from build123d import *

# Parameters (mm, degrees)
F0_W     = 292.1
F0_H     = 38.1
F1_DEPTH = 1219.2
F3_DEPTH = 1219.2
F4_W     = 12.7
F4_H     = 50.8
F5_DEPTH = 254


with BuildPart() as f1:
    # F0 (on Front) → F1 (new body)
    with BuildSketch(Plane.XZ):
        with Locations((146.05, 19.05)):
            Rectangle(F0_W, F0_H)
    extrude(amount=F1_DEPTH)

    # F2 (on face) → F3 (join)
    with BuildSketch(Plane.XZ.offset(1219.2)):
        with BuildLine():
            ThreePointArc((0, 41.275), (0.929936, 39.029936), (3.175, 38.1))
            Line((3.175, 38.1), (22.225, 38.1))
            ThreePointArc((22.225, 38.1), (24.470064, 39.029936), (25.4, 41.275))
            Line((25.4, 41.275), (25.4, 60.325))
            ThreePointArc((25.4, 60.325), (24.470064, 62.570064), (22.225, 63.5))
            Line((22.225, 63.5), (3.175, 63.5))
            ThreePointArc((3.175, 63.5), (0.929936, 62.570064), (0, 60.325))
            Line((0, 60.325), (0, 41.275))
        make_face()
        with BuildLine():
            ThreePointArc((22.6568, 41.275), (22.530329, 40.969671), (22.225, 40.8432))
            Line((22.225, 40.8432), (3.175, 40.8432))
            ThreePointArc((3.175, 40.8432), (2.869671, 40.969671), (2.7432, 41.275))
            Line((2.7432, 41.275), (2.7432, 60.325))
            ThreePointArc((2.7432, 60.325), (2.869671, 60.630329), (3.175, 60.7568))
            Line((3.175, 60.7568), (22.225, 60.7568))
            ThreePointArc((22.225, 60.7568), (22.530329, 60.630329), (22.6568, 60.325))
            Line((22.6568, 60.325), (22.6568, 41.275))
        make_face(mode=Mode.SUBTRACT)
    extrude(amount=-F3_DEPTH)

    # F4 (on face) → F5 (join)
    with BuildSketch(Plane(origin=(0, 0, 0), x_dir=(1, 0, 0), z_dir=(0, 0, -1))):
        with Locations((95.25, 1193.8)):
            Rectangle(F4_W, F4_H)
        with Locations((234.95, 1193.8)):
            Rectangle(F4_W, F4_H)
        with Locations((95.25, 838.2)):
            Rectangle(F4_W, F4_H)
        with Locations((234.95, 838.2)):
            Rectangle(F4_W, F4_H)
    extrude(amount=F5_DEPTH)


solid = f1.part
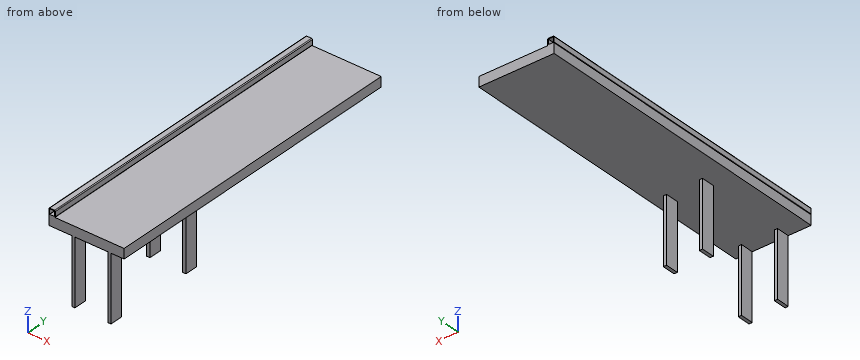
Could you check a few things on this model? Use its own coordinates, in mm. Coordinates: 2 decimals unless noted, no trailing zeros. Write each loop counter-clockwise with the first axis right and the second up, starting at its lowest first coordinate (ties: lowest second). Pieces come first, ordered by that corner, then holes. Notation, with made-up numbers: (24.5, -1) - (40.5, -1) arc R23 cw to (40.5, 18) - close; hole circle Ø2 at (-24.75, 80.5). An arc over 180 degrees is marked (long way). Put each result on its own line as item: value. Start each with the question number.
Q1. I'm going to push flat-ended pins straight in: P1, Ø10, axis at x = 221.5, z = 3, coming from the +Y side; P2, Ø6, axis at x = 95, z = -33, coming from the +Y side; P3, Ø15, axis at y = -838.5, z = -173, coming from the -X side; P4, Ø12, axis at x = 100.5, y = -979, coming from the +Z side. Where does each tip first touch, or does it pass through?
Q2. I want a section at C-C on x = 188.5. Write out the boundary of the cut face in (y, z), plus the area to 3 significant figures.
Q3. I want a section at A-A on z = -177. Write out the boundary of the cut face in (x, y), plus the area to 3 significant figures.
Q4. I want a section at B-B on y = -847. Write out the boundary of the cut face in (x, z) (3 decimals), plus the area to 3 significant figures.
Q5. Please list where these lines run through material, in increasing order: L1, parallel to X at y = -128.5, z = 41; L2, parallel to X at y = -996.5, z = 50.5; L3, parallel to Z at x = 180.5, y = -608.5.
Q6. I want a section at D-D on y = -457.5. Write out the boundary of the cut face in (x, z) (3 decimals), plus the area to 3 significant figures.
Checks:
1. P1: y = 0
1. P2: y = -812.8
1. P3: x = 88.9
1. P4: z = 38.1
2. outline: (-1219.2, 0) - (0, 0) - (0, 38.1) - (-1219.2, 38.1) - close
2. area: 46,500 mm²
3. outline: (88.9, -1219.2) - (101.6, -1219.2) - (101.6, -1168.4) - (88.9, -1168.4) - close; (88.9, -863.6) - (101.6, -863.6) - (101.6, -812.8) - (88.9, -812.8) - close; (228.6, -1219.2) - (241.3, -1219.2) - (241.3, -1168.4) - (228.6, -1168.4) - close; (228.6, -863.6) - (241.3, -863.6) - (241.3, -812.8) - (228.6, -812.8) - close
3. area: 2,580 mm²
4. outline: (0, 0) - (88.9, 0) - (88.9, -254) - (101.6, -254) - (101.6, 0) - (228.6, 0) - (228.6, -254) - (241.3, -254) - (241.3, 0) - (292.1, 0) - (292.1, 38.1) - (22.225, 38.1) arc R3.175 ccw to (25.4, 41.275) - (25.4, 60.325) arc R3.175 ccw to (22.225, 63.5) - (3.175, 63.5) arc R3.175 ccw to (0, 60.325) - (0, 41.275) arc R3.175 ccw to (3.175, 38.1) - (0, 38.1) - close; hole (2.743, 41.275) arc R0.432 ccw to (3.175, 40.843) - (22.225, 40.843) arc R0.432 ccw to (22.657, 41.275) - (22.657, 60.325) arc R0.432 ccw to (22.225, 60.757) - (3.175, 60.757) arc R0.432 ccw to (2.743, 60.325) - close
4. area: 17,800 mm²
5. L1: 0.01 to 2.84, 22.56 to 25.39
5. L2: 0 to 2.74, 22.66 to 25.4
5. L3: 0 to 38.1
6. outline: (0, 0) - (292.1, 0) - (292.1, 38.1) - (22.225, 38.1) arc R3.175 ccw to (25.4, 41.275) - (25.4, 60.325) arc R3.175 ccw to (22.225, 63.5) - (3.175, 63.5) arc R3.175 ccw to (0, 60.325) - (0, 41.275) arc R3.175 ccw to (3.175, 38.1) - (0, 38.1) - close; hole (2.743, 41.275) arc R0.432 ccw to (3.175, 40.843) - (22.225, 40.843) arc R0.432 ccw to (22.657, 41.275) - (22.657, 60.325) arc R0.432 ccw to (22.225, 60.757) - (3.175, 60.757) arc R0.432 ccw to (2.743, 60.325) - close
6. area: 11,400 mm²
